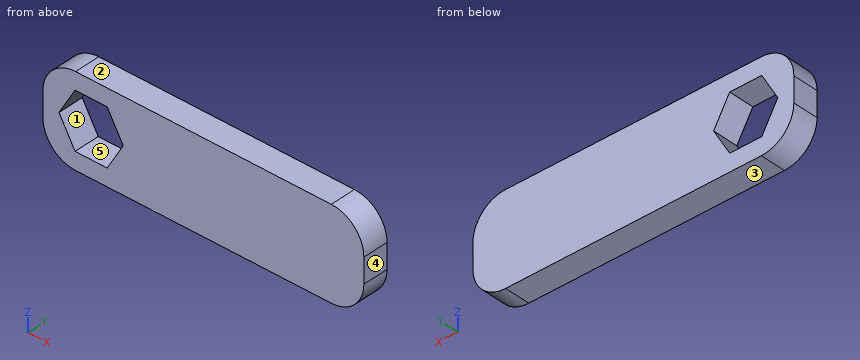
```python
from build123d import *

# Parameters (mm, degrees)
F0_W     = 50
F0_H     = 14
F1_DEPTH = 4
F3_DEPTH = 4.001
F4_R     = 5.08


with BuildPart() as f1:
    # F0 (on Front) → F1 (new body)
    with BuildSketch(Plane.XZ):
        with Locations((25, 7)):
            Rectangle(F0_W, F0_H)
    extrude(amount=F1_DEPTH)

    # F2 (on face) → F3 (cut, through all)
    with BuildSketch(Plane.XZ.offset(4)):
        Polygon((12.5, 7), (10, 11.330127), (5, 11.330127), (2.5, 7), (5, 2.669873), (10, 2.669873), align=None)
    extrude(amount=-F3_DEPTH, mode=Mode.SUBTRACT)

    # F4
    f4_edges = [f1.edges().sort_by_distance(p)[0] for p in [
        (0, -2, 14),
        (50, -2, 14),
        (50, -2, 0),
        (0, -2, 0),
    ]]
    fillet(f4_edges, radius=F4_R)


solid = f1.part
```
Work out the finished part from the listing and answer in its coordinate system (mm). Face numbers are marked on the shaded views. A direction names the side the tool comes from. Give positions to 0.01 mm unless a question says otherwise; leave off trailing zeros. Write each loop counter-clockwise with the first axis right and the second up, starting at its lowest first coordinate (ties: lowest second). Pieces come first, ordered by that corner, then holes. Notation, with made-up numbers: (64, 78) -> (99, 78) arc R15 cw to (99, 107) -> close; hole circle Ø5 at (39, 86). An arc over 180 degrees is marked (long way). Write item = value, one per line.
Q1. For a pull along X with two mould halves and no side action, classify the marked faces 3, 4 and 5 as pulls with the +X half, pulls with the -X half, needs draft (parallel to the pull), parting line crosses it, or undercut.
Computed values:
face_3 = needs draft
face_4 = pulls with the +X half
face_5 = undercut
Q2. A flat-ended cylindrical pin translates along its axis: pin 1 Ø1 at (x, z) = (27, 12) entering from +Y. Find the tip coordinate at first contact, or state that the pin passes through.
Computed values:
pin_1 = 0
Q3. Section A-A on x = 8 is taken. Determine the outline of the cut face in (y, z).
Computed values:
outline = (-4, 0) -> (0, 0) -> (0, 2.67) -> (-4, 2.67) -> close; (-4, 11.33) -> (0, 11.33) -> (0, 14) -> (-4, 14) -> close
Q4. Section D-D on z = 12 is taken. Determine the outline of the cut face in (x, y).
Computed values:
outline = (1.04, -4) -> (48.96, -4) -> (48.96, 0) -> (1.04, 0) -> close
Q5. Section C-C on z = 5.5 is taken. Determine the outline of the cut face in (x, y), and give its area (3 significant figures).
Computed values:
outline = (0, -4) -> (3.37, -4) -> (3.37, 0) -> (0, 0) -> close; (11.63, -4) -> (50, -4) -> (50, 0) -> (11.63, 0) -> close
area = 167 mm^2
Q6. A tool of negligible diameter and unlimited length cuts with its end or side. For the marked faces 1 and 2, from which of +Z, -Z, +X, -X, +Y, -Y can it reach the whole face along a straight path? Write none if from no direction.
Computed values:
face_1 = +Y, -Y
face_2 = +Z, +X, -X, +Y, -Y
Q7. Consider line 1 along Z through (x, y) = (9, -3.5); line 2 along X through (y, z) = (-1.25, 4); line 3 along X through (y, z) = (-0.9, 8.5). Determine where each line is inside the solid, lowest interval first.
Computed values:
line_1 = 0 to 2.67, 11.33 to 14
line_2 = 0.12 to 4.23, 10.77 to 49.88
line_3 = 0 to 3.37, 11.63 to 50
Q8. Section B-B on y = -0.6 is taken. Determine the outline of the cut face in (x, z).
Computed values:
outline = (0, 5.08) arc R5.08 ccw to (5.08, 0) -> (44.92, 0) arc R5.08 ccw to (50, 5.08) -> (50, 8.92) arc R5.08 ccw to (44.92, 14) -> (5.08, 14) arc R5.08 ccw to (0, 8.92) -> close; hole (2.5, 7) -> (5, 2.67) -> (10, 2.67) -> (12.5, 7) -> (10, 11.33) -> (5, 11.33) -> close
